from build123d import *

# Parameters (mm, degrees)
ESQUISSE1_W                                   = 30
ESQUISSE1_H                                   = 26
ESQUISSE1_R                                   = 11.5
BOSS_EXTRU_1_DEPTH                            = 6
ESQUISSE2_R                                   = 12
ENL_V_MAT_EXTRU_1_DEPTH                       = 5
TROU_POUR_TARAUDAGE_POUR_TROU_TARAUD_M2_D     = 1.6
TROU_POUR_TARAUDAGE_POUR_TROU_TARAUD_M2_DEPTH = 5
TROU_POUR_TARAUDAGE_POUR_TROU_TARAUD_M2_TIP   = 0.480688495
TROU_POUR_TARAUDAGE_POUR_TROU_TARAUD_2_D      = 1.6
TROU_POUR_TARAUDAGE_POUR_TROU_TARAUD_2_DEPTH  = 5
TROU_POUR_TARAUDAGE_POUR_TROU_TARAUD_2_TIP    = 0.480688495


with BuildPart() as part:
    # Esquisse1 → Boss.-Extru.1 (new body)
    with BuildSketch(Plane.XY):
        with Locations((15, 13)):
            Rectangle(ESQUISSE1_W, ESQUISSE1_H)
        with Locations((15, 13)):
            Circle(ESQUISSE1_R, mode=Mode.SUBTRACT)
    extrude(amount=BOSS_EXTRU_1_DEPTH)

    # Esquisse2 → Enlèv. mat.-Extru.1 (cut)
    with BuildSketch(Plane.XY.offset(6)):
        with Locations((15, 13)):
            Circle(ESQUISSE2_R)
    extrude(amount=-ENL_V_MAT_EXTRU_1_DEPTH, mode=Mode.SUBTRACT)

    # Trou pour taraudage pour trou taraud_ M2
    with Locations(Plane(origin=(0, 26, 0), x_dir=(1, 0, 0), z_dir=(0, 1, 0))):
        with Locations((4, -3), (26, -3)):
            Hole(TROU_POUR_TARAUDAGE_POUR_TROU_TARAUD_M2_D / 2, depth=TROU_POUR_TARAUDAGE_POUR_TROU_TARAUD_M2_DEPTH)
            with Locations((0, 0, -(TROU_POUR_TARAUDAGE_POUR_TROU_TARAUD_M2_DEPTH + TROU_POUR_TARAUDAGE_POUR_TROU_TARAUD_M2_TIP / 2))):  # 118° drill point
                Cone(0, TROU_POUR_TARAUDAGE_POUR_TROU_TARAUD_M2_D / 2, TROU_POUR_TARAUDAGE_POUR_TROU_TARAUD_M2_TIP, mode=Mode.SUBTRACT)

    # Trou pour taraudage pour trou taraud 2
    with Locations(Plane(origin=(0, 0, 0), x_dir=(-1, 0, 0), z_dir=(0, -1, 0))):
        with Locations((-4, -3), (-26, -3)):
            Hole(TROU_POUR_TARAUDAGE_POUR_TROU_TARAUD_2_D / 2, depth=TROU_POUR_TARAUDAGE_POUR_TROU_TARAUD_2_DEPTH)
            with Locations((0, 0, -(TROU_POUR_TARAUDAGE_POUR_TROU_TARAUD_2_DEPTH + TROU_POUR_TARAUDAGE_POUR_TROU_TARAUD_2_TIP / 2))):  # 118° drill point
                Cone(0, TROU_POUR_TARAUDAGE_POUR_TROU_TARAUD_2_D / 2, TROU_POUR_TARAUDAGE_POUR_TROU_TARAUD_2_TIP, mode=Mode.SUBTRACT)


solid = part.part
Design review of the part built by this model. Coordinates are the model's own, in mm. A direction names the side the tool comes from. Coordinates: 2 decimals unless noted, no trailing zeros. Order: outer loops, then holes, each group sorted by start corner. A loop starts at its lowest first (then second) coordinate and runs counter-clockwise, first axis right, second up. Notation, with made-up numbers: (-29.75, 33.5) - (-18.75, 33.5) arc R37 ccw to (-18.75, 69.5) - close; hole circle Ø10 at (21.25, 50.25). An arc over 180 degrees is marked (long way). Put each result on its own line as item: value.
1) Insertion check: P1, Ø2, axis at x = 6, y = 20, coming from the -Z side; P2, Ø1.4, axis at x = 26, z = 3, coming from the +Y side; P3, Ø5, axis at x = 18.5, y = 21, coming from the +Z side. Each pin has a flat end and moves straight along its axis. Give the tip position at first contact, or say it passes through.
Response values:
P1: stops at z = 0
P2: stops at y = 20.94
P3: passes through
2) Wall thickness on L1, parallel to Z at x = 26, y = 23.9; L2, parallel to Y at x = 15, z = 0.4; L3, parallel to X at y = 2.5, z = 2.4: over which ranges is each line inside the solid? List them lowest first. Write a range as from..to.
Response values:
L1: z = 0..2.2, 3.8..6
L2: y = 0..1.5, 24.5..26
L3: x = 0..3.47, 4.53..9.19, 20.81..25.47, 26.53..30
3) Take a section at B-B, the plane x = 15. Give the boundary of the cut face in (y, z).
Response values:
outline: (0, 0) - (1.5, 0) - (1.5, 1) - (1, 1) - (1, 6) - (0, 6) - close; (24.5, 0) - (26, 0) - (26, 6) - (25, 6) - (25, 1) - (24.5, 1) - close
4) The part is to be moulded in two halves that separate along X. For faces 6 (the face through (15, 0, 3)), 7 (the face through (4.8, 23.5, 3)), 8 (the face through (30, 13, 3)), say which applies: released by +X, released by -X, zero draft, split by the parting line, or undercut.
Response values:
face 6: zero draft
face 7: undercut
face 8: released by +X
5) Take a section at D-D, the plane z = 0.65. Give the boundary of the cut face in (x, y).
Response values:
outline: (0, 0) - (30, 0) - (30, 26) - (0, 26) - close; hole circle Ø23 at (15, 13)
6) Tool access review of faces 1 (the face through (6.156, 21.11, 3.535)), 2 (the face through (25.237, 23.465, 2.76)), 3 (the face through (5, 19, 0)), 4 (the face through (0, 13, 3)), 5 (the face through (3.37, 2.54, 3.49)): name each direction out of +Z, -Z, +X, -X, +Y, -Y from which nothing blocks a thin tool from reaching the whole face with its end or side.
Response values:
face 1: +Z
face 2: +Y
face 3: -Z, +X, -X, +Y, -Y
face 4: +Z, -Z, -X, +Y, -Y
face 5: -Y
7) Take a section at C-C, the plane z = 5.1. Give the boundary of the cut face in (x, y).
Response values:
outline: (0, 0) - (30, 0) - (30, 26) - (0, 26) - close; hole circle Ø24 at (15, 13)
8) Take a section at A-A, the plane y = 13. Give the boundary of the cut face in (x, z).
Response values:
outline: (0, 0) - (3.5, 0) - (3.5, 1) - (3, 1) - (3, 6) - (0, 6) - close; (26.5, 0) - (30, 0) - (30, 6) - (27, 6) - (27, 1) - (26.5, 1) - close
